Could you check a few things on this model? Use its own coordinates, in mm. Coordinates: 2 decimals unless noted, no trailing zeros. Loops run counter-clockwise (first coordinate to the right, second up) from the corner with the lowest first, then second, coordinate; pieces in that order, holes last.
1) If I drill on line 1 along X through (y, z) = (0.2, 51.5); line 2 along Z through (x, y) = (-48, 0.2); line 3 along X through (y, z) = (0.1, -44), over which ranges is the centre line in solid material (lowest first)?
2) Imagine slicing it at A-A on y = 0.1. Please give me the cut outline in (x, z).
3) Imagine slicing it at B-B on z = -32. Please give me the cut outline in (x, y) (3 decimals).
4) Imagine slicing it at C-C on x = 51.5. Please give me the cut outline in (y, z), plus the area to 3 significant figures.
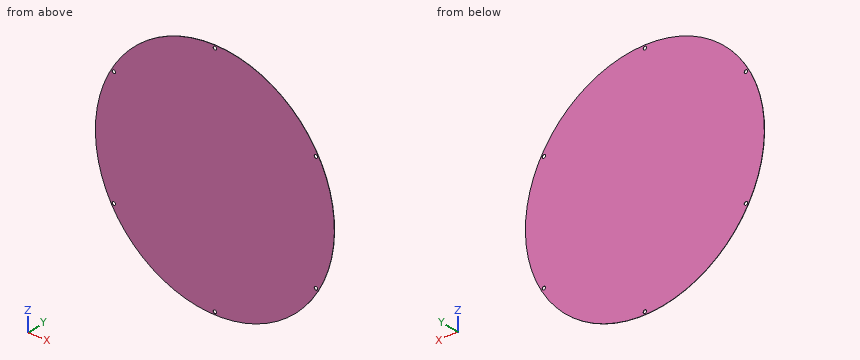
```python
from build123d import *

# Parameters (mm, degrees)
SKETCH1_R           = 105
SKETCH1_R_2         = 1.4732
SKETCH1_R_3         = 100
BOSS_EXTRUDE1_DEPTH = 0.254


with BuildPart() as part:
    # Sketch1 → Boss-Extrude1 (new body)
    # profile 1 of 2: a face of its own
    with BuildSketch(Plane(origin=(0, 0, 0), x_dir=(1, 0, 0), z_dir=(0, 1, 0))):
        with Locations(Location((0, 0, 0), (0, 0, 270))):
            Circle(SKETCH1_R)
        with Locations(Location((88.768103888, -51.250866025, 0), (0, 0, 270))):
            Circle(SKETCH1_R_2, mode=Mode.SUBTRACT)
        with Locations(Location((88.769103888, 51.249133975, 0), (0, 0, 270))):
            Circle(SKETCH1_R_2, mode=Mode.SUBTRACT)
        with Locations(Location((0.002, 102.5, 0), (0, 0, 270))):
            Circle(SKETCH1_R_2, mode=Mode.SUBTRACT)
        with Locations(Location((-88.766103888, 51.250866025, 0), (0, 0, 270))):
            Circle(SKETCH1_R_2, mode=Mode.SUBTRACT)
        with Locations(Location((-88.767103888, -51.249133975, 0), (0, 0, 270))):
            Circle(SKETCH1_R_2, mode=Mode.SUBTRACT)
        with Locations(Location((0, -102.5, 0), (0, 0, 270))):
            Circle(SKETCH1_R_2, mode=Mode.SUBTRACT)
        Circle(SKETCH1_R_3, mode=Mode.SUBTRACT)
    # profile 2 of 2: a face of its own
    with BuildSketch(Plane(origin=(0, 0, 0), x_dir=(1, 0, 0), z_dir=(0, 1, 0))):
        Circle(SKETCH1_R_3)
    extrude(amount=BOSS_EXTRUDE1_DEPTH)


solid = part.part
```
Filled in:
1. line 1: x = -91.5 to -90.22, -87.32 to 87.32, 90.22 to 91.5
1. line 2: z = -93.39 to 93.39
1. line 3: x = -95.34 to 95.34
2. outline: circle Ø210 at (0, 0); hole circle Ø2.95 at (-88.77, -51.25); hole circle Ø2.95 at (-88.77, 51.25); hole circle Ø2.95 at (0, -102.5); hole circle Ø2.95 at (0, 102.5); hole circle Ø2.95 at (88.77, 51.25); hole circle Ø2.95 at (88.77, -51.25)
3. outline: (-100.005, 0) - (100.005, 0) - (100.005, 0.254) - (-100.005, 0.254) - close
4. outline: (0, -91.5) - (0.25, -91.5) - (0.25, 91.5) - (0, 91.5) - close
4. area: 46.5 mm2
